For this review, use the dimensioned drawing (mm, ordinates from the lowest corner) and the shaded views. Round coordinates to 2 decimals unless told otherwise and drop trailing zeros. Write each loop counter-clockwise with the first axis right and the second up, starting at its lowest first coordinate (ties: lowest second). Pieces come first, ordered by that corner, then holes. Notation, with made-up numbers: M 50.5,84 L 62.5,84 A14 cw 62.5,97 Z; hole C 58.5,-31.5 d1. An arc over 180 degrees is marked long. One line per question, with ' | ' between items. Start each with the question number.
Item 1: Insertion check: pin 1 Ø8 at (x, y) = (14.5, 15.5) entering from +Z; pin 2 Ø3 at (y, z) = (26, 5) entering from +X; pin 3 Ø3 at (y, z) = (6, 5) entering from -X; pin 4 Ø2 at (y, z) = (26, 15) entering from -X. Each pin has a flat end and moves straight along its axis. Give the tip position at first contact, or say it passes through.
Item 2: Add section B-B, the plane y = 18. State the section outline as (x, z) points.
Item 3: Add section C-C, the plane x = 15.75. State the section outline as (y, z) points (1 decimal).
Item 4: Add section A-A, the plane z = 11.5. State the section outline as (x, y) points.
Item 5: Draft analysis for pull direction Z (two halves, no side actions). For the marked faces 1, 2 and 3, state which applies: released by +Z, released by -Z, zero draft, split by the parting line, or undercut.
Item 6: For L1, parallel to Z at x = 3, y = 26; L2, parallel to Y at x = 22, z = 15; L3, parallel to X at y = 16, z = 13.5, list the stretches that pass through material, from the lowest coordinate up.
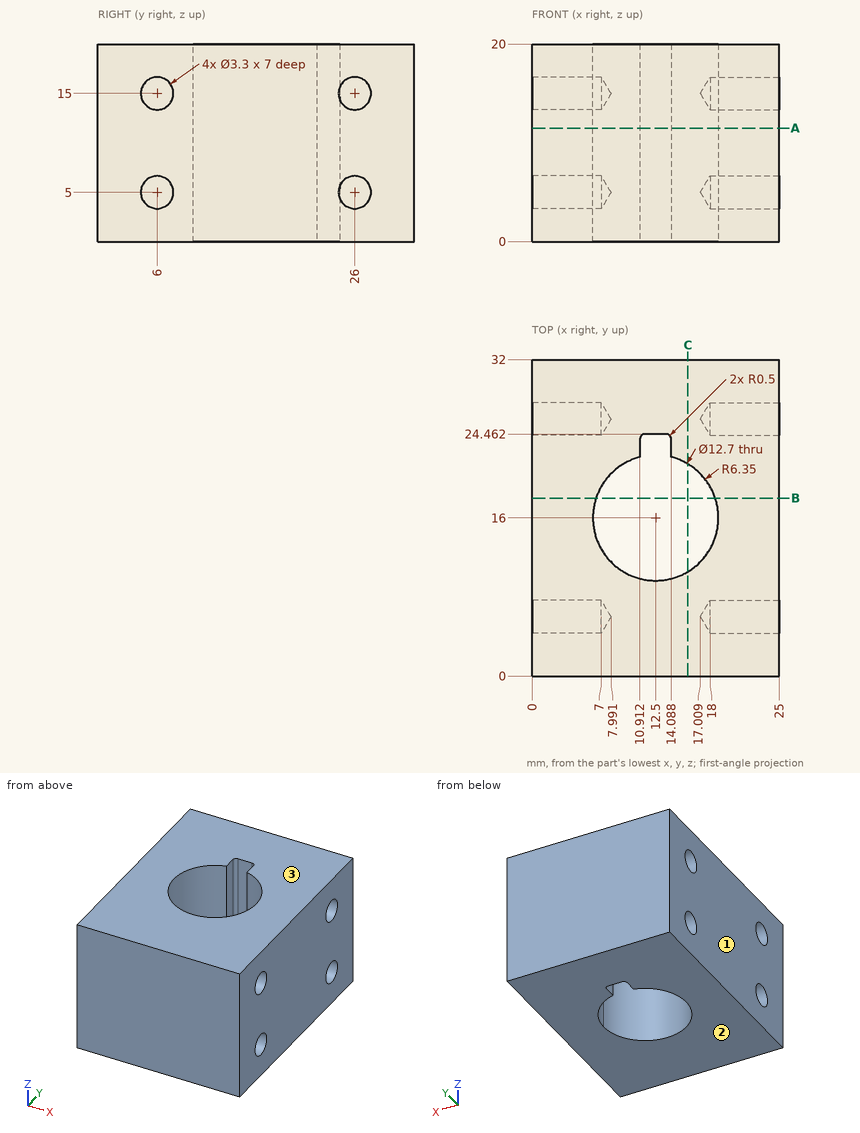
Computed values:
1) pin 1: passes through | pin 2: stops at x = 17.91 | pin 3: stops at x = 7.09 | pin 4: stops at x = 7.39
2) outline: M 0,0 L 6.47,0 L 6.47,20 L 0,20 Z; M 18.53,0 L 25,0 L 25,20 L 18.53,20 Z
3) outline: M 0,0 L 10.5,0 L 10.5,20 L 0,20 Z; M 21.5,0 L 32,0 L 32,20 L 21.5,20 Z
4) outline: M 0,0 L 25,0 L 25,32 L 0,32 Z; hole M 10.91,22.15 A6.35 ccw long 14.09,22.15 L 14.09,23.96 A0.5 ccw 13.59,24.46 L 11.41,24.46 A0.5 ccw 10.91,23.96 Z
5) face 1: zero draft | face 2: released by -Z | face 3: released by +Z
6) L1: z = 0 to 3.35, 6.65 to 13.35, 16.65 to 20 | L2: y = 0 to 4.35, 7.65 to 24.35, 27.65 to 32 | L3: x = 0 to 6.15, 18.85 to 25
